Check sheet for the modelled part. Datum: model origin and axes. Units: mm. A direction names the side the tool comes from. Give positions to 0.01 mm unless a question says otherwise; leave off trailing zeros. Order: outer loops, then holes, each group sorted by start corner. A loop starts at its lowest first (then second) coordinate and runs counter-clockwise, first axis right, second up.
```python
from build123d import *

# Parameters (mm, degrees)
SKETCH2_R          = 3
CUT_EXTRUDE1_DEPTH = 23


with BuildPart() as part:
    # Sketch1 → Revolve1 (revolve)
    with BuildSketch(Plane.XY):
        Polygon((8.827160494, 15.308641975), (18.827160494, 15.308641975), (18.827160494, 5.308641975), (13.827160494, -4.691358025), (3.827160494, -4.691358025), (3.827160494, 5.308641975), (8.827160494, 5.308641975), align=None)
    revolve(axis=Axis((-1.172839506, 0, 0), (0, 1, 0)))

    # Sketch2 → Cut-Extrude1 (cut)
    with BuildSketch(Plane.XY):
        with Locations((0, 10.308641975)):
            Circle(SKETCH2_R)
    extrude(amount=-CUT_EXTRUDE1_DEPTH, mode=Mode.SUBTRACT)


solid = part.part
```
Q1. Draft check along Y on faces 1 (the flat face through (-3, 5.309, -5)), 2 (the flat face through (-5, -4.691, -4)), 3 (the cylindrical face through (2.86, 11.21, -14.47)). Enter one of: pulls with the +Y half, pulls with the -Y half, needs draft (parallel to the pull), parting line crosses it, or undercut.
Q2. Material ranges on line 1 (X direction, y = 12.75, z = 0); line 2 (Z direction, x = -3, y = 6); line 3 (Z direction, x = -2.5, y = 12.75), recorded low to high.
Q3. Sectioned sample at C-C, the plane x = 0. Count the separate pieces of the cut face and the enclosed holes in it, plus the area to 3 significant figures.
Q4. Tool access check on faces 4 (the flat face through (4, 15.309, -9)), 5 (the cylindrical face through (-3.341, 10.379, 9.762)). Record the directions out of +Z, -Z, +X, -X, +Y, -Y that give a thin tool (end or side, any length) a straight path to the whole face; none if there is none.
Q5. Sectioned sample at A-A, the plane z = 0. Record the cut outline in (x, y).
Q6. Sectioned sample at D-D, the plane y = 0. Record the cut outline in (x, z), plus the area to 3 significant figures.
Q7. Go/stop test with flat-tipped pins: P1, Ø5.5, axis at x = 0, y = 10.31, coming from the -Z side; P2, Ø6, axis at x = 1.5, y = 1.5, coming from the -Z side; P3, Ø10, axis at x = 6, y = 13, coming from the +Z side; P4, Ø10, axis at x = 6.5, z = 0, coming from the +Y side. Record where each tip stops, or that it passes through.
Q8. Sectioned sample at B-B, the plane y = 6.5. Record the cut outline in (x, z).
Filled in:
1. face 1: pulls with the +Y half
1. face 2: pulls with the -Y half
1. face 3: undercut
2. line 1: x = -21.17 to -11.17, 8.83 to 18.83
2. line 2: z = -19.92 to -9.83, 9.83 to 19.92
2. line 3: z = -19.96 to -9.91, 9.91 to 19.96
3. separate pieces: 3
3. enclosed holes: 0
3. area: 392 mm2
4. face 4: +Z, -Z, +X, -X, +Y
4. face 5: +Y
5. outline: (-21.17, 5.31) - (-16.17, -4.69) - (-6.17, -4.69) - (-6.17, 5.31) - (-11.17, 5.31) - (-11.17, 15.31) - (-21.17, 15.31) - close; (3.83, -4.69) - (13.83, -4.69) - (18.83, 5.31) - (18.83, 15.31) - (8.83, 15.31) - (8.83, 5.31) - (3.83, 5.31) - close
6. outline: circle Ø34.69 at (-1.17, 0); hole circle Ø10 at (-1.17, 0)
6. area: 867 mm2
7. P1: stops at z = 9.2
7. P2: stops at z = -19.46
7. P3: stops at z = 19.88
7. P4: stops at y = 15.31
8. outline: circle Ø40 at (-1.17, 0); hole circle Ø20 at (-1.17, 0)
